Here's how the part is built. I have some questions about the finished solid (model axes, mm). A direction names the side the tool comes from. Round coordinates to 2 decimals unless told otherwise and drop trailing zeros. Write each loop counter-clockwise with the first axis right and the second up, starting at its lowest first coordinate (ties: lowest second). Pieces come first, ordered by that corner, then holes. Notation, with made-up numbers: (17, 58) - (68, 58) arc R29 cw to (68, 93) - close; hole circle Ø7 at (53, 21). An arc over 180 degrees is marked (long way). One line per item, written item: value. Start each with the question number.
Item 1: Imagine slicing it at D-D, the plane z = 7.25. Please give me the cut outline in (x, y), then the cut area to 3 significant figures.
Item 2: For P1, Ø12, axis at x = -14.5, y = 18, coming from the +Z side; P2, Ø4, axis at y = 0, z = 4, coming from the -X side; P3, Ø1.5, axis at x = -13.5, y = -2.5, coming from the -Z side, each with a flat end and sliding along its axis, tell me the tip position at first contact or that it passes through.
Item 3: Imagine slicing it at C-C, the plane z = 12. Please give me the cut outline in (x, y), then the cut area to 3 significant figures.
Item 4: Imagine slicing it at B-B, the plane y = 27.5. Please give me the cut outline in (x, z), then the cut area to 3 significant figures.
Item 5: For faces 1 (the face through (0, 0, -2)), 2 (the face through (15.5, -2, 7)), 3 (the face through (-10.5, -2, 7)), 4 (the face through (-5, 9, -2)), which set-ups out of +Z, -Z, +X, -X, +Y, -Y let a thin tool reach every point of the face, with its end or its side?
Item 6: Imagine slicing it at A-A, the plane z = -1.25. Please give me the cut outline in (x, y), then the cut area to 3 significant figures.
Item 7: If I drill on line 1 (Z direction, x = -14.1, y = -7); line 2 (X direction, y = -4, z = 12.75); line 3 (Z direction, x = -16, y = 1), over which ranges is the centre line in solid material (lowest first)?
Autodesk Inventor part; units mm, degrees
ref_plane "작업 평면1" through (10.5, 0, 0) normal (1, 0, 0) x (0, 1, 0)
ref_plane "XZ Plane" through (0, 0, 0) normal (0, 1, 0) x (-1, 0, 0)
ref_plane "XY Plane" through (0, 0, 0) normal (0, 0, 1) x (1, 0, 0)
sketch "스케치1" plane through (0, 0, 0) normal (0, 0, 1) x (1, 0, 0)
  line L0 (0, 0) -> (0, 40)
  line L1 (0, 0) -> (40, 0) construction
  line L2 (0, 0) -> (-21, 0)
  line L3 (-15.3431, 14) -> (-5, 14)
  line L4 (-5, 14) -> (-5, 4)
  line L5 (-5, 4) -> (0, 4)
  line L6 (-21, 0) -> (-21, 14)
  line L7 (-21, 14) -> (0, 35)
  line L8 (-15.3431, 14) -> (0, 29.3431)
  line L9 (0, 0) -> (21, 0)
  line L10 (15.3431, 14) -> (5, 14)
  line L11 (5, 14) -> (5, 4)
  line L12 (5, 4) -> (0, 4)
  line L13 (21, 0) -> (21, 14)
  line L14 (21, 14) -> (0, 35)
  line L15 (15.3431, 14) -> (0, 29.3431)
  dimension "d0" = 40
  dimension "d2" = 35
  dimension "d3" = 4
  dimension "d4" = 10
  dimension "d6" = 42
  dimension "d8" = 4
  dimension "d9" = 10
  dimension "d10" = 45
extrude "돌출1" add sketch "스케치1" against normal blind 4 contours L2 L6 L7 L0 L8 L3 L4 L5 | L0 L12 L11 L10 L15 L14 L13 L9
ref_plane "작업 평면1" through (10.5, 0, 0) normal (1, 0, 0) x (0, 1, 0)
sketch "스케치3" plane through (10.5, 0, 0) normal (1, 0, 0) x (0, 1, 0)
  circle A0 centre (-7, 8) radius 3
  arc A1 (-7, 14) -> (-7, 2) centre (-7, 8) ccw
  line L0 (14, 0) -> (0, 0)
  line L1 (9, 0) -> (1, 14)
  line L2 (1, 14) -> (-7, 14)
  line L3 (0, 0) -> (0, -4)
  line L4 (0, 0) -> (0, 2)
  line L5 (0, 2) -> (-7, 2)
  dimension "d14" = 6
  dimension "d15" = 12
  dimension "d16" = 8
  dimension "d17" = 8
  dimension "d18" = 6
  dimension "d19" = 12
  dimension "d20" = 14
  dimension "d21" = 7
extrude "돌출2" add sketch "스케치3" along normal blind 5
mirror "미러1" about plane through (0, 0, 0) normal (1, 0, 0) of "돌출2"
fillet "모깎기1" radius 2 4 edges at (-21, 14, -2) (-21, 0, -2) (21, 14, -2) (21, 0, -2)
properties part number "01-1"
Values follow:
1. outline: (-15.5, -12.95) - (-10.5, -12.95) - (-10.5, -9.9) - (-15.5, -9.9) - close; (-15.5, -4.1) - (-10.5, -4.1) - (-10.5, 4.86) - (-15.5, 4.86) - close; (10.5, -12.95) - (15.5, -12.95) - (15.5, -9.9) - (10.5, -9.9) - close; (10.5, -4.1) - (15.5, -4.1) - (15.5, 4.86) - (10.5, 4.86) - close
1. area: 120 mm^2
2. P1: stops at z = 0
2. P2: stops at x = -15.5
2. P3: stops at z = 2
3. outline: (-15.5, -11.47) - (-10.5, -11.47) - (-10.5, 2.14) - (-15.5, 2.14) - close; (10.5, -11.47) - (15.5, -11.47) - (15.5, 2.14) - (10.5, 2.14) - close
3. area: 136 mm^2
4. outline: (-7.5, -4) - (-1.84, -4) - (-1.84, 0) - (-7.5, 0) - close; (1.84, -4) - (7.5, -4) - (7.5, 0) - (1.84, 0) - close
4. area: 45.3 mm^2
5. face 1: -Z, +X, -X, -Y
5. face 2: +Z, +X, +Y, -Y
5. face 3: +Z, +Y, -Y
5. face 4: +Z, -Z
6. outline: (-21, 2) arc R2 ccw to (-19, 0) - (19, 0) arc R2 ccw to (21, 2) - (21, 13.17) arc R2 ccw to (20.41, 14.59) - (0, 35) - (-20.41, 14.59) arc R2 ccw to (-21, 13.17) - close; hole (-15.34, 14) - (-5, 14) - (-5, 4) - (5, 4) - (5, 14) - (15.34, 14) - (0, 29.34) - close
6. area: 692 mm^2
7. line 1: z = 2 to 5, 11 to 14
7. line 2: x = -15.5 to -10.5, 10.5 to 15.5
7. line 3: z = -4 to 0
